from build123d import *

# Parameters (mm, degrees)
MODEL_R                 = 1.5
MODEL_W                 = 3
MODEL_H                 = 3
SALIENTE_EXTRUIR1_DEPTH = 3


with BuildPart() as part:
    # Model → Saliente-Extruir1 (new body)
    with BuildSketch(Plane.XY):
        with BuildLine():
            Line((17.356035274, 193.902048875), (53.356035274, 193.902048875))
            ThreePointArc((53.356035274, 193.902048875), (56.53801579, 195.22006836), (57.856035274, 198.402048875))
            Line((57.856035274, 198.402048875), (57.856035274, 288.402048875))
            ThreePointArc((57.856035274, 288.402048875), (56.53801579, 291.58402939), (53.356035274, 292.902048875))
            Line((53.356035274, 292.902048875), (17.356035274, 292.902048875))
            ThreePointArc((17.356035274, 292.902048875), (14.174054759, 291.58402939), (12.856035274, 288.402048875))
            Line((12.856035274, 288.402048875), (12.856035274, 198.402048875))
            ThreePointArc((12.856035274, 198.402048875), (14.174054759, 195.22006836), (17.356035274, 193.902048875))
        make_face()
        with Locations((40.355847758, 226.651825621)):
            Circle(MODEL_R, mode=Mode.SUBTRACT)
        with Locations((30.355847768, 226.652272077)):
            Circle(MODEL_R, mode=Mode.SUBTRACT)
        with Locations((40.358013069, 275.151825573)):
            Circle(MODEL_R, mode=Mode.SUBTRACT)
        with Locations((30.35801308, 275.152272029)):
            Circle(MODEL_R, mode=Mode.SUBTRACT)
        with Locations((53.356035274, 288.402048875)):
            Rectangle(MODEL_W, MODEL_H, mode=Mode.SUBTRACT)
        with Locations((53.356035274, 279.402048875)):
            Rectangle(MODEL_W, MODEL_H, mode=Mode.SUBTRACT)
        with Locations((53.356035274, 270.402048875)):
            Rectangle(MODEL_W, MODEL_H, mode=Mode.SUBTRACT)
        with Locations((53.356035274, 261.402048875)):
            Rectangle(MODEL_W, MODEL_H, mode=Mode.SUBTRACT)
        with Locations((53.356035274, 252.402048875)):
            Rectangle(MODEL_W, MODEL_H, mode=Mode.SUBTRACT)
        with Locations((53.356035274, 243.402048875)):
            Rectangle(MODEL_W, MODEL_H, mode=Mode.SUBTRACT)
        with Locations((53.356035274, 234.402048875)):
            Rectangle(MODEL_W, MODEL_H, mode=Mode.SUBTRACT)
        with Locations((53.356035274, 225.402048875)):
            Rectangle(MODEL_W, MODEL_H, mode=Mode.SUBTRACT)
        with Locations((53.356035274, 216.402048875)):
            Rectangle(MODEL_W, MODEL_H, mode=Mode.SUBTRACT)
        with Locations((53.356035274, 207.402048875)):
            Rectangle(MODEL_W, MODEL_H, mode=Mode.SUBTRACT)
        with Locations((53.356035274, 198.402048875)):
            Rectangle(MODEL_W, MODEL_H, mode=Mode.SUBTRACT)
        with Locations((17.356035274, 288.402048875)):
            Rectangle(MODEL_W, MODEL_H, mode=Mode.SUBTRACT)
        with Locations((17.356035274, 279.402048875)):
            Rectangle(MODEL_W, MODEL_H, mode=Mode.SUBTRACT)
        with Locations((17.356035274, 270.402048875)):
            Rectangle(MODEL_W, MODEL_H, mode=Mode.SUBTRACT)
        with Locations((17.356035274, 261.402048875)):
            Rectangle(MODEL_W, MODEL_H, mode=Mode.SUBTRACT)
        with Locations((17.356035274, 252.402048875)):
            Rectangle(MODEL_W, MODEL_H, mode=Mode.SUBTRACT)
        with Locations((17.356035274, 243.402048875)):
            Rectangle(MODEL_W, MODEL_H, mode=Mode.SUBTRACT)
        with Locations((17.356035274, 234.402048875)):
            Rectangle(MODEL_W, MODEL_H, mode=Mode.SUBTRACT)
        with Locations((17.356035274, 225.402048875)):
            Rectangle(MODEL_W, MODEL_H, mode=Mode.SUBTRACT)
        with Locations((17.356035274, 216.402048875)):
            Rectangle(MODEL_W, MODEL_H, mode=Mode.SUBTRACT)
        with Locations((17.356035274, 207.402048875)):
            Rectangle(MODEL_W, MODEL_H, mode=Mode.SUBTRACT)
        with Locations((17.356035274, 198.402048875)):
            Rectangle(MODEL_W, MODEL_H, mode=Mode.SUBTRACT)
        with Locations((44.356035274, 198.402048875)):
            Rectangle(MODEL_W, MODEL_H, mode=Mode.SUBTRACT)
        with Locations((26.356035274, 198.402048875)):
            Rectangle(MODEL_W, MODEL_H, mode=Mode.SUBTRACT)
        with Locations((35.356035274, 198.402048875)):
            Rectangle(MODEL_W, MODEL_H, mode=Mode.SUBTRACT)
        with Locations((44.356035274, 216.402048875)):
            Rectangle(MODEL_W, MODEL_H, mode=Mode.SUBTRACT)
        with Locations((26.356035274, 216.402048875)):
            Rectangle(MODEL_W, MODEL_H, mode=Mode.SUBTRACT)
        with Locations((35.356035274, 216.402048875)):
            Rectangle(MODEL_W, MODEL_H, mode=Mode.SUBTRACT)
        with Locations((44.356035274, 207.402048875)):
            Rectangle(MODEL_W, MODEL_H, mode=Mode.SUBTRACT)
        with Locations((26.356035274, 207.402048875)):
            Rectangle(MODEL_W, MODEL_H, mode=Mode.SUBTRACT)
        with Locations((35.356035274, 207.402048875)):
            Rectangle(MODEL_W, MODEL_H, mode=Mode.SUBTRACT)
        with Locations((44.356035274, 288.402048875)):
            Rectangle(MODEL_W, MODEL_H, mode=Mode.SUBTRACT)
        with Locations((26.356035274, 288.402048875)):
            Rectangle(MODEL_W, MODEL_H, mode=Mode.SUBTRACT)
        with Locations((35.356035274, 288.402048875)):
            Rectangle(MODEL_W, MODEL_H, mode=Mode.SUBTRACT)
        with Locations((44.356035274, 279.402048875)):
            Rectangle(MODEL_W, MODEL_H, mode=Mode.SUBTRACT)
        with Locations((26.356035274, 279.402048875)):
            Rectangle(MODEL_W, MODEL_H, mode=Mode.SUBTRACT)
        with BuildLine():
            Line((33.857854573, 280.901620206), (33.857854573, 276.931747225))
            ThreePointArc((33.857854573, 276.931747225), (33.491829169, 276.565721821), (33.357854573, 276.065721821))
            Line((33.357854573, 276.065721821), (33.357854573, 272.401620206))
            ThreePointArc((33.357854573, 272.401620206), (33.010514208, 271.827023537), (32.378058676, 271.601620206))
            Line((32.378058676, 271.601620206), (25.757854573, 271.601620206))
            ThreePointArc((25.757854573, 271.601620206), (25.404597365, 271.455492569), (25.25783227, 271.102499725))
            Line((25.25783227, 271.102499725), (25.25756379, 265.088924432))
            ThreePointArc((25.25756379, 265.088924432), (22.355834382, 256.902629272), (25.256832814, 248.716075046))
            Line((25.256832814, 248.716075046), (25.256057607, 231.352499765))
            ThreePointArc((25.256057607, 231.352499765), (25.402488432, 230.998939836), (25.756035284, 230.852477443))
            Line((25.756035284, 230.852477443), (34.556035275, 230.852084561))
            Line((34.556035275, 230.852084561), (34.555724988, 223.902084568))
            Line((34.555724988, 223.902084568), (36.155724986, 223.902013135))
            Line((36.155724986, 223.902013135), (36.156035273, 230.852013128))
            Line((36.156035273, 230.852013128), (44.956035265, 230.851620247))
            ThreePointArc((44.956035265, 230.851620247), (45.309595193, 230.998051072), (45.456057587, 231.351597924))
            Line((45.456057587, 231.351597924), (45.456832945, 248.718539377))
            ThreePointArc((45.456832945, 248.718539377), (48.355834356, 256.901468487), (45.45756362, 265.084656419))
            Line((45.45756362, 265.084656419), (45.45783225, 271.101597884))
            ThreePointArc((45.45783225, 271.101597884), (45.311401425, 271.455157812), (44.957854573, 271.601620206))
            Line((44.957854573, 271.601620206), (38.33765047, 271.601620206))
            ThreePointArc((38.33765047, 271.601620206), (37.705194938, 271.827023537), (37.357854573, 272.401620206))
            Line((37.357854573, 272.401620206), (37.357854573, 276.065721821))
            ThreePointArc((37.357854573, 276.065721821), (37.223879977, 276.565721821), (36.857854573, 276.931747225))
            Line((36.857854573, 276.931747225), (36.857854573, 280.901620206))
            Line((36.857854573, 280.901620206), (33.857854573, 280.901620206))
        make_face(mode=Mode.SUBTRACT)
    extrude(amount=SALIENTE_EXTRUIR1_DEPTH)


solid = part.part
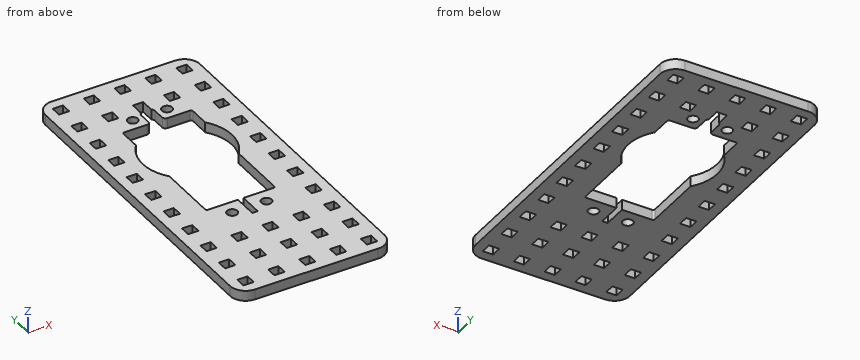
CAD build for the part. Positions are in the model's coordinates, mm. Coordinates: 2 decimals unless noted, no trailing zeros. Write each loop counter-clockwise with the first axis right and the second up, starting at its lowest first coordinate (ties: lowest second). Pieces come first, ordered by that corner, then holes. Notation, with made-up numbers: M -39,73.25 L -11,73.25 A19 ccw -11,87.25 Z; hole C 3.5,-30.5 d5. An arc over 180 degrees is marked long. Return JSON: item names as keys, results as strings.
Item 1: Slice it at A-A, the plane y = 217. Write the cut outline in (x, z), and give its area (3 significant figures).
Findings below:
{"outline": "M 12.86,0 L 15.86,0 L 15.86,3 L 12.86,3 Z; M 18.86,0 L 24.86,0 L 24.86,3 L 18.86,3 Z; M 27.86,0 L 33.86,0 L 33.86,3 L 27.86,3 Z; M 36.86,0 L 42.86,0 L 42.86,3 L 36.86,3 Z; M 45.86,0 L 51.86,0 L 51.86,3 L 45.86,3 Z; M 54.86,0 L 57.86,0 L 57.86,3 L 54.86,3 Z", "area": "90.0 mm2"}
Item 2: Probe line 1 (X direction, y = 199, z = 1); line 2 (X direction, y = 270.5, z = 0.6); line 3 (Y direction, x = 34, z = 1.05). List the from-to ranges inside material, lowest first. Write a range as from..to.
Findings below:
{"line 1": "x = 12.86..15.86, 18.86..24.86, 27.86..33.86, 36.86..42.86, 45.86..51.86, 54.86..57.86", "line 2": "x = 12.86..15.86, 18.86..25.26, 45.46..51.86, 54.86..57.86", "line 3": "y = 193.9..196.9, 199.9..205.9, 208.9..214.9, 217.9..230.85, 280.9..286.9, 289.9..292.9"}
Item 3: Drop flat-ended pins along their axis: pin 1 Ø1 at (x, y) = (40, 215) entering from -Z; pin 2 Ø0.9 at (x, z) = (54, 1.5) entering from +Y. Give the stop position or say it passes through.
Findings below:
{"pin 1": "stops at z = 0", "pin 2": "stops at y = 292.9"}
Item 4: Slice it at C-C, the plane z = 1.7. State how many separate pieces and enclosed holes the cut face has, and give its area (3 significant figures).
Findings below:
{"separate pieces": "1", "enclosed holes": "41", "area": "3,150 mm2"}
Item 5: Slice it at B-B, the plane y = 270. Write the cut outline in (x, z), and give its area (3 significant figures).
Findings below:
{"outline": "M 12.86,0 L 15.86,0 L 15.86,3 L 12.86,3 Z; M 18.86,0 L 25.26,0 L 25.26,3 L 18.86,3 Z; M 45.46,0 L 51.86,0 L 51.86,3 L 45.46,3 Z; M 54.86,0 L 57.86,0 L 57.86,3 L 54.86,3 Z", "area": "56.4 mm2"}
